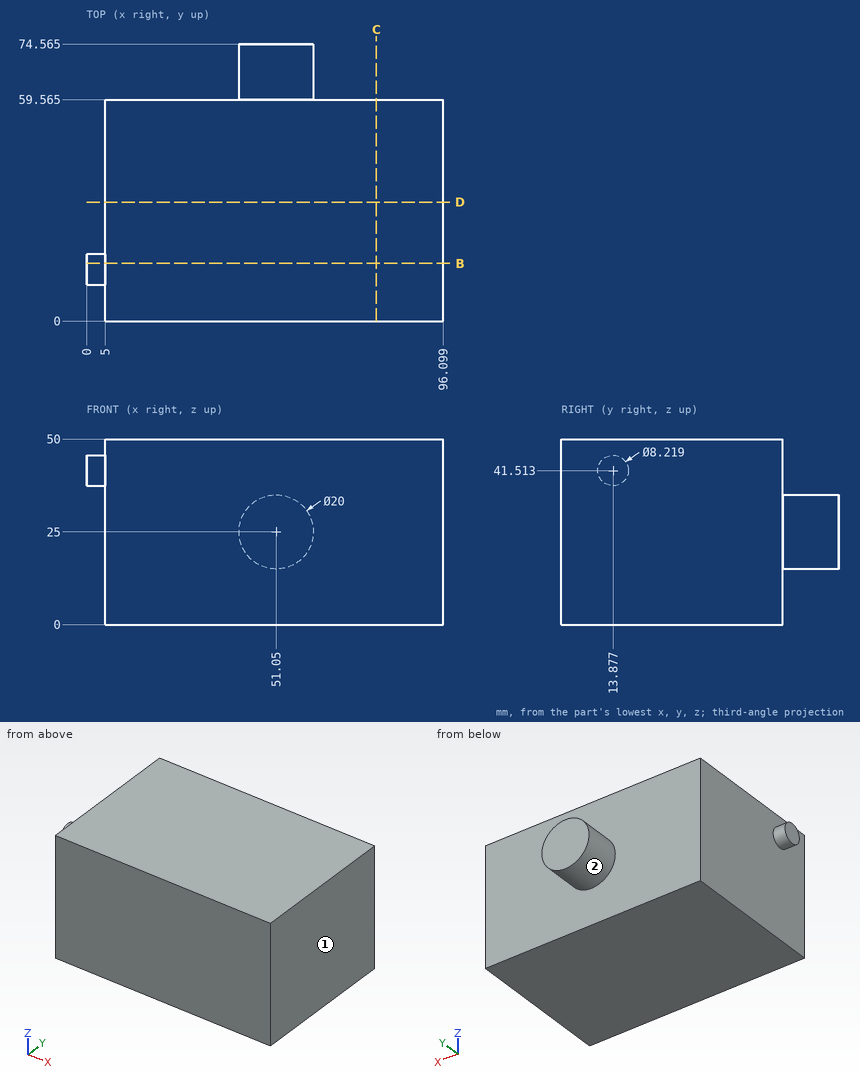
Verification items for this drawing (mm, ordinates from the low corner). A direction names the side the tool comes from. Coordinates: 2 decimals unless noted, no trailing zeros. Write each loop counter-clockwise with the first axis right and the second up, starting at its lowest first coordinate (ties: lowest second). Pieces come first, ordered by that corner, then holes. Notation, with made-up numbers: M -19.75,34 L -11.75,34 A27 cw -11.75,63 Z; hole C 69.25,-31.5 d1. An arc over 180 degrees is marked long. Answer as a JSON object with one key per item and string values.
1. Tool access check on the marked faces 1 and 2. Record the directions out of +Z, -Z, +X, -X, +Y, -Y that give a thin tool (end or side, any length) a straight path to the whole face; none if there is none.
Answers below:
{"face 1": "+Z, -Z, +X, +Y, -Y", "face 2": "+Y"}
2. Scan lines: L1, parallel to Y at x = 8.5, z = 42 (1 decimal); L2, parallel to X at y = 3, z = 40.5; L3, parallel to X at y = 68, z = 26. Record each from-to range of solid material in increasing order.
Answers below:
{"L1": "y = 0 to 59.6", "L2": "x = 5 to 96.1", "L3": "x = 41.1 to 61"}
3. Section check D-D, the plane y = 32. Enter the section's corners in (x, z), plus the area to 4 significant figures.
Answers below:
{"outline": "M 5,0 L 96.1,0 L 96.1,50 L 5,50 Z", "area": "4,555 mm²"}
4. Go/stop test with flat-tipped pins: pin 1 Ø6 at (x, y) = (71, 9.5) entering from -Z; pin 2 Ø10 at (x, z) = (25.5, 27.5) entering from +Y (3 decimals); pin 3 Ø1.5 at (y, z) = (55.5, 22) entering from -X. Record where each tip stops, or that it passes through.
Answers below:
{"pin 1": "stops at z = 0", "pin 2": "stops at y = 59.565", "pin 3": "stops at x = 5"}
5. Section check B-B, the plane y = 15.5. Enter the section's corners in (x, z).
Answers below:
{"outline": "M 0,37.74 L 5,37.74 L 5,0 L 96.1,0 L 96.1,50 L 5,50 L 5,45.29 L 0,45.29 Z"}
6. Section check C-C, the plane x = 78. Enter the section's corners in (y, z) (1 decimal), plus the area to 3 significant figures.
Answers below:
{"outline": "M 0,0 L 59.6,0 L 59.6,50 L 0,50 Z", "area": "2,980 mm²"}
